The listing builds one solid part. Answer for the finished solid, in the listing's coordinates (mm). Face numbers are marked on the shaded views. A direction names the side the tool comes from. Give positions to 0.01 mm unless a question says otherwise; leave off trailing zeros. Write each loop counter-clockwise with the first axis right and the second up, starting at its lowest first coordinate (ties: lowest second). Pieces come first, ordered by that corner, then holes. Notation, with made-up numbers: M -24,10 L 19,10 A27 cw 19,48 Z; hole C 34.5,62.25 d2. An arc over 180 degrees is marked long. Answer as a JSON object with one key per item and string values.
```python
from build123d import *

# Parameters (mm, degrees)
BOSS_EXTRUDE1_DEPTH = 8.76
BOSS_EXTRUDE2_START = -0.95
BOSS_EXTRUDE2_DEPTH = 0.95
SKETCH4_W           = 12.8
SKETCH4_H           = 6.9
CUT_EXTRUDE1_DEPTH  = 8
SKETCH5_W           = 1.3986406
SKETCH5_H           = 2.263006611
BOSS_EXTRUDE3_DEPTH = 7.81
CUT_EXTRUDE2_DEPTH  = 8
FILLET1_R           = 0.5
SKETCH8_W           = 8.94
SKETCH8_H           = 3.85
CUT_EXTRUDE6_DEPTH  = 8
FILLET2_R           = 1.28
BOSS_EXTRUDE5_START = 1.9
BOSS_EXTRUDE5_DEPTH = 1.9
CHAMFER1_SIZE       = 0.7
SKETCH14_R          = 1.6
CUT_EXTRUDE10_DEPTH = 6
SKETCH16_R          = 1.6
CUT_EXTRUDE11_DEPTH = 6
CUT_EXTRUDE12_DEPTH = 0.9
SKETCH19_W          = 7.7
SKETCH19_H          = 3.35
CUT_EXTRUDE13_DEPTH = 4
CHAMFER2_SIZE       = 0.5
FILLET3_R           = 0.4


with BuildPart() as part:
    # Sketch1 → Boss-Extrude1 (new body)
    with BuildSketch(Plane(origin=(0, 0, 0), x_dir=(1, 0, 0), z_dir=(0, 1, 0))):
        with BuildLine():
            ThreePointArc((0, 3), (0.878679656, 0.878679656), (3, 0))
            Line((3, 0), (73, 0))
            ThreePointArc((73, 0), (75.121320344, 0.878679656), (76, 3))
            Line((76, 3), (76, 55.62))
            Line((76, 55.62), (76, 57.326548644))
            Line((76, 57.326548644), (76, 61.882562509))
            ThreePointArc((76, 61.882562509), (75.121320344, 64.003882853), (73, 64.882562509))
            Line((73, 64.882562509), (3, 64.882562509))
            ThreePointArc((3, 64.882562509), (0.878679656, 64.003882853), (0, 61.882562509))
            Line((0, 61.882562509), (0, 57.326548644))
            Line((0, 57.326548644), (0, 55.62))
            Line((0, 55.62), (0, 3))
        make_face()
        with BuildLine():
            Line((65, 4), (11, 4))
            ThreePointArc((11, 4), (8.878679656, 4.878679656), (8, 7))
            Line((8, 7), (8, 53.326548644))
            ThreePointArc((8, 53.326548644), (8.878679656, 55.447868988), (11, 56.326548644))
            Line((11, 56.326548644), (65, 56.326548644))
            ThreePointArc((65, 56.326548644), (67.121320344, 55.447868988), (68, 53.326548644))
            Line((68, 53.326548644), (68, 7))
            ThreePointArc((68, 7), (67.121320344, 4.878679656), (65, 4))
        make_face(mode=Mode.SUBTRACT)
    extrude(amount=BOSS_EXTRUDE1_DEPTH)

    # Sketch2 → Boss-Extrude2 (add)
    with BuildSketch(Plane(origin=(0, 8.76, 0), x_dir=(1, 0, 0), z_dir=(0, 1, 0)).offset(BOSS_EXTRUDE2_START)):
        with BuildLine():
            Line((8, 48.62), (8, 7))
            ThreePointArc((8, 7), (8.878679656, 4.878679656), (11, 4))
            Line((11, 4), (65, 4))
            ThreePointArc((65, 4), (67.121320344, 4.878679656), (68, 7))
            Line((68, 7), (68, 48.62))
            Line((68, 48.62), (68, 53.326548644))
            ThreePointArc((68, 53.326548644), (67.121320344, 55.447868988), (65, 56.326548644))
            Line((65, 56.326548644), (11, 56.326548644))
            ThreePointArc((11, 56.326548644), (8.878679656, 55.447868988), (8, 53.326548644))
            Line((8, 53.326548644), (8, 48.62))
        make_face()
    extrude(amount=BOSS_EXTRUDE2_DEPTH)

    # Sketch4 → Cut-Extrude1 (cut)
    with BuildSketch(Plane.ZY):
        with Locations((-28.14, 3.45)):
            Rectangle(SKETCH4_W, SKETCH4_H)
    extrude(amount=-CUT_EXTRUDE1_DEPTH, mode=Mode.SUBTRACT)

    # Sketch5 → Boss-Extrude3 (add)
    with BuildSketch(Plane.XZ):
        with Locations((8.6993203, -20.608496695)):
            Rectangle(SKETCH5_W, SKETCH5_H)
        with Locations((8.6993203, -35.671503305)):
            Rectangle(SKETCH5_W, SKETCH5_H)
    extrude(amount=-BOSS_EXTRUDE3_DEPTH)

    # Sketch6 → Cut-Extrude2 (cut)
    with BuildSketch(Plane(origin=(76, 0, 0), x_dir=(0, 0, -1), z_dir=(1, 0, 0))):
        with BuildLine():
            Line((12.55338903, 2.34), (12.55338903, 0))
            Line((12.55338903, 0), (23.359580852, 0))
            Line((23.359580852, 0), (23.359580852, 2.34))
            ThreePointArc((23.359580852, 2.34), (23.154555599, 2.834974747), (22.659580852, 3.04))
            Line((22.659580852, 3.04), (13.25338903, 3.04))
            ThreePointArc((13.25338903, 3.04), (12.758414283, 2.834974747), (12.55338903, 2.34))
        make_face()
    extrude(amount=-CUT_EXTRUDE2_DEPTH, mode=Mode.SUBTRACT)

    # Fillet1
    fillet1_edges = [part.edges().sort_by_distance(p)[0] for p in [
        (4, 6.9, -34.54),
        (4, 6.9, -21.74),
    ]]
    fillet(fillet1_edges, radius=FILLET1_R)

    # Sketch8 → Cut-Extrude6 (cut)
    with BuildSketch(Plane(origin=(76, 0, 0), x_dir=(0, 0, -1), z_dir=(1, 0, 0))):
        with Locations((29.64, 1.925)):
            Rectangle(SKETCH8_W, SKETCH8_H)
    extrude(amount=-CUT_EXTRUDE6_DEPTH, mode=Mode.SUBTRACT)

    # Fillet2
    fillet2_edges = [part.edges().sort_by_distance(p)[0] for p in [
        (72, 3.85, -34.11),
        (72, 3.85, -25.17),
    ]]
    fillet(fillet2_edges, radius=FILLET2_R)

    # Sketch9 → Boss-Extrude5 (add)
    with BuildSketch(Plane.ZY.offset(-68).offset(BOSS_EXTRUDE5_START)):
        with BuildLine():
            Line((-34.11, 0.47), (-34.11, 2.57))
            ThreePointArc((-34.11, 2.57), (-33.73509668, 3.47509668), (-32.83, 3.85))
            Line((-32.83, 3.85), (-26.45, 3.85))
            ThreePointArc((-26.45, 3.85), (-25.54490332, 3.47509668), (-25.17, 2.57))
            Line((-25.17, 2.57), (-25.17, 0.47))
            Line((-25.17, 0.47), (-24.52, 0.47))
            Line((-24.52, 0.47), (-24.52, 2.57))
            ThreePointArc((-24.52, 2.57), (-25.085283912, 3.934716088), (-26.45, 4.5))
            Line((-26.45, 4.5), (-32.83, 4.5))
            ThreePointArc((-32.83, 4.5), (-34.194716088, 3.934716088), (-34.76, 2.57))
            Line((-34.76, 2.57), (-34.76, 0.47))
            Line((-34.76, 0.47), (-34.11, 0.47))
        make_face()
    extrude(amount=-BOSS_EXTRUDE5_DEPTH)

    # Chamfer1
    chamfer1_edges = [part.edges().sort_by_distance(p)[0] for p in [
        (76, 1.17, -23.359580852),
        (76, 2.834974747, -23.154555599),
        (76, 3.04, -17.956484941),
        (76, 2.834974747, -12.758414283),
        (76, 1.17, -12.55338903),
        (76, 1.285, -34.11),
        (76, 3.85, -29.64),
        (76, 1.285, -25.17),
        (76, 3.47509668, -33.73509668),
        (76, 3.47509668, -25.54490332),
    ]]
    chamfer(chamfer1_edges, length=CHAMFER1_SIZE)

    # Sketch14 → Cut-Extrude10 (cut)
    with BuildSketch(Plane(origin=(0, 0, 0), x_dir=(-1, 0, 0), z_dir=(0, -1, 0))):
        with Locations(Location((-4.7, 6, 0), (0, 0, 90))):
            Circle(SKETCH14_R)
        with Locations(Location((-4.7, 58.885125018, 0), (0, 0, 270))):
            Circle(SKETCH14_R)
    extrude(amount=-CUT_EXTRUDE10_DEPTH, mode=Mode.SUBTRACT)

    # Sketch16 → Cut-Extrude11 (cut)
    with BuildSketch(Plane(origin=(0, 0, 0), x_dir=(-1, 0, 0), z_dir=(0, -1, 0))):
        with Locations(Location((-71.3, 6, 0), (0, 0, 90))):
            Circle(SKETCH16_R)
        with Locations(Location((-71.3, 58.88, 0), (0, 0, 270))):
            Circle(SKETCH16_R)
    extrude(amount=-CUT_EXTRUDE11_DEPTH, mode=Mode.SUBTRACT)

    # Sketch18 → Cut-Extrude12 (cut)
    with BuildSketch(Plane(origin=(0, 0, -64.882562509), x_dir=(-1, 0, 0), z_dir=(0, 0, -1))):
        with BuildLine():
            Line((-64.583936573, -0.08), (-11.416063427, -0.08))
            Line((-11.416063427, -0.08), (-11.42000005, 2.410060225))
            ThreePointArc((-11.42000005, 2.410060225), (-11.704466584, 3.096728386), (-12.391153239, 3.381150275))
            Line((-12.391153239, 3.381150275), (-38.000003545, 3.38))
            Line((-38.000003545, 3.38), (-63.608843072, 3.381150275))
            ThreePointArc((-63.608843072, 3.381150275), (-64.295532112, 3.096729691), (-64.57999995, 2.410060225))
            Line((-64.57999995, 2.410060225), (-64.583936573, -0.08))
        make_face()
    extrude(amount=-CUT_EXTRUDE12_DEPTH, mode=Mode.SUBTRACT)

    # Sketch19 → Cut-Extrude13 (cut)
    with BuildSketch(Plane.XY):
        with Locations((30.53, 1.675)):
            Rectangle(SKETCH19_W, SKETCH19_H)
    extrude(amount=-CUT_EXTRUDE13_DEPTH, mode=Mode.SUBTRACT)

    # Chamfer2
    chamfer2_edges = [part.edges().sort_by_distance(p)[0] for p in [
        (34.38, 3.35, -2),
        (26.68, 3.35, -2),
    ]]
    chamfer(chamfer2_edges, length=CHAMFER2_SIZE)

    # Fillet3
    fillet3_edges = [part.edges().sort_by_distance(p)[0] for p in [
        (27.18, 3.35, -2),
        (33.88, 3.35, -2),
        (34.38, 2.85, -2),
        (26.68, 2.85, -2),
    ]]
    fillet(fillet3_edges, radius=FILLET3_R)


solid = part.part
```
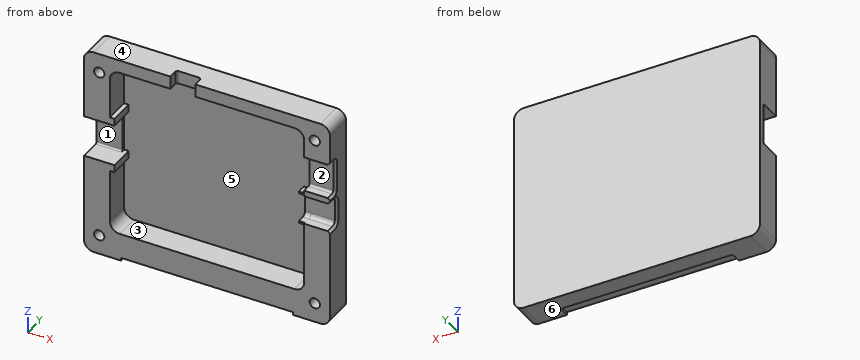
1. A cutting plane is placed at C-C, the plane z = -11. Give the vertices of the cut face in (x, y).
Verdict:
{"outline": "M 0,0 L 8,0 L 8,7.81 L 68,7.81 L 68,0 L 76,0 L 76,8.76 L 0,8.76 Z"}
2. Consider line 1 along Z through (x, y) = (71.3, 4.8); line 2 along X through (y, z) = (3.25, -51); line 3 along Z through (x, y) = (71.3, 2.9). Determine where each line is inside the solid, lowest interval first.
Verdict:
{"line 1": "z = -64.88 to -60.48, -57.28 to -7.6, -4.4 to 0", "line 2": "x = 0 to 8, 68 to 76", "line 3": "z = -64.88 to -60.48, -57.28 to -34.07, -25.21 to -23.08, -12.83 to -7.6, -4.4 to 0"}
3. Flat-ended cylindrical pins translate along their axes: pin 1 (4 mm diameter, centred on x = 51.5, z = -44, fed in from -Y); pin 2 (1 mm diameter, centred on x = 35.5, y = 1, fed in from -Z); pin 3 (4 mm diameter, centred on x = 5, z = -29, fed in from -Y). Find the tip coordinate at first contact, or state that the pin passes through.
Verdict:
{"pin 1": "stops at y = 7.81", "pin 2": "stops at z = -63.98", "pin 3": "stops at y = 6.9"}
4. A cutting plane is placed at D-D, the plane x = 4.7. Give the vertices of the cut face in (y, z).
Verdict:
{"outline": "M 0,-64.88 L 8.76,-64.88 L 8.76,0 L 0,0 L 0,-4.4 L 6,-4.4 L 6,-7.6 L 0,-7.6 L 0,-21.74 L 6.4,-21.74 A0.5 cw 6.9,-22.24 L 6.9,-34.04 A0.5 cw 6.4,-34.54 L 0,-34.54 L 0,-57.29 L 6,-57.29 L 6,-60.49 L 0,-60.49 Z"}
5. For the marked faces 1, 2 and 3, determine the directions among +Z, -Z, +X, -X, +Y, -Y from which every point of the face is accessible in a straight line to the end or side of a thin tool.
Verdict:
{"face 1": "-X, -Y", "face 2": "+X, -Y", "face 3": "-Y"}
6. The mould has two halves that part along Z. Classify the marked faces 4, 5 and 6: released by +Z, released by -Z, zero draft, split by the parting line, or undercut.
Verdict:
{"face 4": "released by +Z", "face 5": "undercut", "face 6": "released by -Z"}
7. A cutting plane is placed at B-B, the plane x = 71.3. Give the vertices of the cut face in (y, z).
Verdict:
{"outline": "M 0,-64.88 L 8.76,-64.88 L 8.76,0 L 0,0 L 0,-4.4 L 6,-4.4 L 6,-7.6 L 0,-7.6 L 0,-12.55 L 2.34,-12.55 A0.7 cw 3.04,-13.25 L 3.04,-22.66 A0.7 cw 2.34,-23.36 L 0,-23.36 L 0,-25.17 L 2.57,-25.17 A1.28 cw 3.85,-26.45 L 3.85,-32.83 A1.28 cw 2.57,-34.11 L 0,-34.11 L 0,-57.28 L 6,-57.28 L 6,-60.48 L 0,-60.48 Z"}
8. A cutting plane is placed at A-A, the plane z = -28. Give the vertices of the cut face in (x, y).
Verdict:
{"outline": "M 0,6.9 L 8,6.9 L 8,7.81 L 68,7.81 L 68,4.5 L 66.1,4.5 L 66.1,3.85 L 75.3,3.85 L 76,4.55 L 76,8.76 L 0,8.76 Z"}
